```python
from build123d import *

# Parameters (mm, degrees)
SKETCH1_R           = 1.1176
BOSS_EXTRUDE1_DEPTH = 5.08
SKETCH2_R           = 1.0922
CUT_EXTRUDE1_DEPTH  = 15.748
SKETCH3_W           = 8.001
SKETCH3_H           = 5.08
SKETCH3_R           = 2.131785714
CUT_EXTRUDE2_DEPTH  = 15.748


with BuildPart() as part:
    # Sketch1 → Boss-Extrude1 (new body)
    with BuildSketch(Plane.XY):
        with BuildLine():
            Line((4.0005, -21.59), (4.0005, 1.368360053))
            ThreePointArc((4.0005, 1.368360053), (0, 4.228050317), (-4.0005, 1.368360053))
            Line((-4.0005, 1.368360053), (-4.0005, -21.59))
            Line((-4.0005, -21.59), (4.0005, -21.59))
        make_face()
        Circle(SKETCH1_R, mode=Mode.SUBTRACT)
    extrude(amount=BOSS_EXTRUDE1_DEPTH)

    # Sketch2 → Cut-Extrude1 (cut)
    with BuildSketch(Plane.XZ.offset(21.59)):
        with Locations(Location((0, 2.54, 0), (0, 0, 270))):
            Circle(SKETCH2_R)
    extrude(amount=-CUT_EXTRUDE1_DEPTH, mode=Mode.SUBTRACT)

    # Sketch3 → Cut-Extrude2 (cut)
    with BuildSketch(Plane.XZ.offset(21.59)):
        with Locations((0, 2.54)):
            Rectangle(SKETCH3_W, SKETCH3_H)
        with Locations(Location((0, 2.54, 0), (0, 0, 270))):
            Circle(SKETCH3_R, mode=Mode.SUBTRACT)
    extrude(amount=-CUT_EXTRUDE2_DEPTH, mode=Mode.SUBTRACT)


solid = part.part
```
Check sheet for the modelled part. Datum: model origin and axes. Units: mm. A direction names the side the tool comes from. Coordinates: 2 decimals unless noted, no trailing zeros. Order: outer loops, then holes, each group sorted by start corner. A loop starts at its lowest first (then second) coordinate and runs counter-clockwise, first axis right, second up. Notation, with made-up numbers: (31.5, 2) -> (90.5, 2) arc R18 ccw to (90.5, 12) -> close; hole circle Ø11 at (50, 33.5). An arc over 180 degrees is marked (long way). Write item = value, one per line. Start each with the question number.
1) Cross-section at B-B (y = 0). Enter the section's corners in (x, z).
2) Cross-section at D-D (z = 4.1). Enter the section's corners in (x, y).
3) Mould release check, pull along Y, two halves, no side actions. Record for faces 3 (the flat face through (0, -5.842, 3)), 4 (the cylindrical face through (0.073, 4.227, 2.504)), 5 (the flat face through (4, -2, 3)), 6 (the cylindrical face through (-0.887, -0.68, 2.504)): +Y half, -Y half, draft (parallel to the pull), parting line (faces both ways), or undercut.
4) Go/stop test with flat-tipped pins: P1, Ø0.7, axis at x = 0.5, z = 3, coming from the -Y side; P2, Ø3, axis at x = -1.5, y = -8.5, coming from the -Z side. Record where each tip stops, or that it passes through.
5) Material ranges on L1, parallel to Y at x = 0, z = 1.2; L2, parallel to Y at x = 0, z = 1.7; L3, parallel to X at y = -14, z = 2.54, recorded low to high.
6) Cross-section at A-A (x = 0). Enter the section's corners in (y, z), then the cut area to 3 significant figures.
7) Access from +Z, -Z, +X, -X, +Y, -Y to the whole of each face (thin tool, end or side, straight path). Record for faces 1 (the flat face through (0, -2, 0)), 2 (the cylindrical face through (0.05, -13.83, 3.63)).
8) Cross-section at C-C (z = 2.54). Enter the section's corners in (x, y), then the cut area to 3 significant figures.
Ans:
q1.outline = (-4, 0) -> (-1.12, 0) -> (-1.12, 5.08) -> (-4, 5.08) -> close; (1.12, 0) -> (4, 0) -> (4, 5.08) -> (1.12, 5.08) -> close
q2.outline = (-4, -5.84) -> (-1.45, -5.84) -> (-1.45, -21.59) -> (1.45, -21.59) -> (1.45, -5.84) -> (4, -5.84) -> (4, 1.37) arc R4.23 ccw to (-4, 1.37) -> close; hole circle Ø2.24 at (0, 0)
q3.face_3 = -Y half
q3.face_4 = +Y half
q3.face_5 = draft
q3.face_6 = undercut
q4.P1 = -5.84
q4.P2 = 0.41
q5.L1 = -21.59 to -1.12, 1.12 to 4.23
q5.L2 = -5.84 to -1.12, 1.12 to 4.23
q5.L3 = -2.13 to -1.09, 1.09 to 2.13
q6.outline = (-21.59, 0.41) -> (-5.84, 0.41) -> (-5.84, 0) -> (-1.12, 0) -> (-1.12, 5.08) -> (-5.84, 5.08) -> (-5.84, 4.67) -> (-21.59, 4.67) -> (-21.59, 3.63) -> (-5.84, 3.63) -> (-5.84, 1.45) -> (-21.59, 1.45) -> close; (1.12, 0) -> (4.23, 0) -> (4.23, 5.08) -> (1.12, 5.08) -> close
q6.area = 72.5 mm²
q7.face_1 = -Z, +X, -X, +Y, -Y
q7.face_2 = -Y
q8.outline = (-4, -5.84) -> (-2.13, -5.84) -> (-2.13, -21.59) -> (-1.09, -21.59) -> (-1.09, -5.84) -> (1.09, -5.84) -> (1.09, -21.59) -> (2.13, -21.59) -> (2.13, -5.84) -> (4, -5.84) -> (4, 1.37) arc R4.23 ccw to (-4, 1.37) -> close; hole circle Ø2.24 at (0, 0)
q8.area = 103 mm²
